The listing builds one solid part. Answer for the finished solid, in the listing's coordinates (mm). A direction names the side the tool comes from. Coordinates: 2 decimals unless noted, no trailing zeros. Order: outer loops, then holes, each group sorted by start corner. A loop starts at its lowest first (then second) coordinate and runs counter-clockwise, first axis right, second up. Notation, with made-up numbers: (47, 89) -> (90, 89) arc R18 ccw to (90, 109) -> close; hole circle Ø2 at (25, 5.25). An arc over 180 degrees is marked (long way). Write item = value, one per line. Start each with the question number.
```python
from build123d import *

# Parameters (mm, degrees)
SKETCH1_R           = 1.651
BOSS_EXTRUDE1_DEPTH = 79.756
SKETCH3_R           = 6.858
CUT_EXTRUDE2_DEPTH  = 67.056
CUT_EXTRUDE3_DEPTH  = 12.7


with BuildPart() as part:
    # Sketch1 → Boss-Extrude1 (new body)
    with BuildSketch(Plane(origin=(0, 0, 0), x_dir=(1, 0, 0), z_dir=(0, 1, 0))):
        with BuildLine():
            ThreePointArc((-46.347101967, -12.820550524), (-45.953093742, -7.978326418), (-45.607903753, -3.132377527))
            ThreePointArc((-45.607903753, -3.132377527), (-43.324155634, 14.457824244), (-38.846810395, 31.621276211))
            ThreePointArc((-38.846810395, 31.621276211), (-38.301804917, 33.429574735), (-37.849619012, 35.263287481))
            ThreePointArc((-37.849619012, 35.263287481), (-28.512474187, 39.785530688), (-26.300260653, 29.649502453))
            ThreePointArc((-26.300260653, 29.649502453), (-27.908796698, 27.470225182), (-29.278925969, 25.133692836))
            ThreePointArc((-29.278925969, 25.133692836), (-32.172639115, 18.448511751), (-34.117731608, 11.428409395))
            ThreePointArc((-34.117731608, 11.428409395), (-35.22666999, -0.274420306), (-33.831690761, -11.946609488))
            ThreePointArc((-33.831690761, -11.946609488), (-33.67793303, -13.064327384), (-33.724408967, -14.191613825))
            ThreePointArc((-33.724408967, -14.191613825), (-33.760843575, -16.790093108), (-33.198139816, -19.327175397))
            ThreePointArc((-33.198139816, -19.327175397), (-31.977523501, -22.310967081), (-30.442888304, -25.146070573))
            ThreePointArc((-30.442888304, -25.146070573), (-30.782899932, -28.090653785), (-33.723620439, -28.462596122))
            ThreePointArc((-33.723620439, -28.462596122), (-40.997268986, -22.504520927), (-46.230736135, -14.693282563))
            ThreePointArc((-46.230736135, -14.693282563), (-46.358471746, -13.761238335), (-46.347101967, -12.820550524))
        make_face()
        with Locations((-31.399492492, 33.846007028)):
            Circle(SKETCH1_R, mode=Mode.SUBTRACT)
        with Locations((-40.020695033, -13.367428306)):
            Circle(SKETCH1_R, mode=Mode.SUBTRACT)
    extrude(amount=BOSS_EXTRUDE1_DEPTH)

    # Sketch3 → Cut-Extrude2 (cut)
    with BuildSketch(Plane(origin=(0, 6.35, 0), x_dir=(-1, 0, 0), z_dir=(0, 1, 0))):
        with Locations((31.399492492, -33.846007028)):
            Circle(SKETCH3_R)
        with BuildLine():
            Line((33.192444355, 5.435760509), (47.285899843, 5.435760509))
            Line((47.285899843, 5.435760509), (46.632941201, 11.116111886))
            ThreePointArc((46.632941201, 11.116111886), (46.99317865, 13.785396267), (46.316644417, 16.392531007))
            Line((46.316644417, 16.392531007), (44.60108667, 21.165715919))
            Line((44.60108667, 21.165715919), (30.194900336, 21.165715919))
            Line((30.194900336, 21.165715919), (33.055086417, 12.847311389))
            ThreePointArc((33.055086417, 12.847311389), (33.189965557, 11.90751056), (33.451045025, 10.994682267))
            Line((33.451045025, 10.994682267), (33.192444355, 5.435760509))
        make_face()
    extrude(amount=CUT_EXTRUDE2_DEPTH, mode=Mode.SUBTRACT)

    # Sketch4 → Cut-Extrude3 (cut)
    with BuildSketch(Plane(origin=(0, 6.35, 0), x_dir=(-1, 0, 0), z_dir=(0, 1, 0))):
        Polygon((28.455486036, -25.206679833), (46.063076484, -25.206679833), (52.862178533, 3.477031937), (29.73031767, 3.477031937), align=None)
    extrude(amount=CUT_EXTRUDE3_DEPTH, mode=Mode.SUBTRACT)


solid = part.part
```
Item 1: Which of the six approach directions +Z, -Z, +X, -X, +Y, -Y give full straight-line access (tool end or side, diameter ignored) to faces 3 (the flat face through (-40, 39, 5.436)), 4 (the cylindrical face through (-31.683, 39.32, 22.915)), 5 (the cylindrical face through (-41.67, 3.13, 13.29))?
Item 2: Section A-A, the plane z = 7.5 is taken. Give the vertices of the cut face in (x, y).
Item 3: Section C-C, the plane y = 11.5 is taken. Give the number of separate pieces and of enclosed holes in the cut face, then the cut area to 3 significant figures.
Item 4: Each of these flat-tipped pins is pushed along its axis until it touches: pin 1 (3 mm diameter, centred on x = -31.4, z = -33.85, fed in from +Y); pin 2 (1 mm diameter, centred on x = -43.5, y = 34, fed in from +Z); pin 3 (3 mm diameter, centred on y = 34.5, z = -31.5, fed in from +X); pin 4 (4 mm diameter, centred on x = -28.5, y = 45, fed in from +Z). Where does it stop, or does it pass through?
Item 5: Consider probe 1 along Y at (x, z) = (-42, 17.5); probe 2 along Z at (x, y) = (-37.25, 9); probe 3 along Z at (x, y) = (-37, 8.5). Determine where each line is inside the solid, lowest interval first.
Item 6: For a pull along Y with two mould halves and no side action, classify faces 1 (the cylindrical face through (-34.466, 39.409, -27.712)), 2 (the cylindrical face through (-29, 77, -40)) as pulls with the +Y half, pulls with the -Y half, needs draft (parallel to the pull), parting line crosses it, or undercut.
Item 7: Section B-B, the plane x = -39.75 is taken. Give the vertices of the cut face in (y, z).
A:
q1.face_3 = +X, -X
q1.face_4 = +X, +Y, -Y
q1.face_5 = +Y, -Y
q2.outline = (-45.92, 0) -> (-34.66, 0) -> (-34.66, 6.35) -> (-45.92, 6.35) -> close; (-45.92, 73.41) -> (-34.66, 73.41) -> (-34.66, 79.76) -> (-45.92, 79.76) -> close
q3.separate_pieces = 3
q3.enclosed_holes = 0
q3.area = 115 mm^2
q4.pin_1 = through
q4.pin_2 = 5.44
q4.pin_3 = -37.08
q4.pin_4 = 27.75
q5.probe_1 = 0 to 6.35, 73.41 to 79.76
q5.probe_2 = -30.27 to -25.21, 3.48 to 5.44, 21.17 to 26.02
q5.probe_3 = -29.89 to -25.21, 3.48 to 5.44, 21.17 to 26.22
q6.face_1 = undercut
q6.face_2 = needs draft
q7.outline = (0, -28.78) -> (79.76, -28.78) -> (79.76, 11.74) -> (73.41, 11.74) -> (73.41, 5.44) -> (6.35, 5.44) -> (6.35, 11.74) -> (0, 11.74) -> close; (0, 15) -> (6.35, 15) -> (6.35, 21.17) -> (73.41, 21.17) -> (73.41, 15) -> (79.76, 15) -> (79.76, 23.8) -> (0, 23.8) -> close; hole (6.35, -25.21) -> (19.05, -25.21) -> (19.05, 3.48) -> (6.35, 3.48) -> close
